from build123d import *

# Parameters (mm, degrees)
SKETCH1_R           = 5.499999036
BOSS_EXTRUDE1_DEPTH = 19
SKETCH2_W           = 11
SKETCH2_H           = 19
CUT_EXTRUDE1_DEPTH  = 33
SKETCH3_W           = 7.598245287
SKETCH3_H           = 4.916511656
CUT_EXTRUDE2_DEPTH  = 33


with BuildPart() as part:
    # Sketch1 → Boss-Extrude1 (new body)
    with BuildSketch(Plane(origin=(0, 0, 0), x_dir=(0, 0, -1), z_dir=(1, 0, 0))):
        with BuildLine():
            Line((-1.999999523, 9.000000954), (11.000000477, 9.000000954))
            Line((11.000000477, 9.000000954), (11.000000477, -9.000000954))
            Line((11.000000477, -9.000000954), (-1.999999523, -9.000000954))
            ThreePointArc((-1.999999523, -9.000000954), (-11.000000477, 0), (-1.999999523, 9.000000954))
        make_face()
        with Locations((-1.999999523, 0)):
            Circle(SKETCH1_R, mode=Mode.SUBTRACT)
    extrude(amount=BOSS_EXTRUDE1_DEPTH)

    # Sketch2 → Cut-Extrude1 (cut)
    with BuildSketch(Plane(origin=(0, 9.000000954, 0), x_dir=(1, 0, 0), z_dir=(0, 1, 0))):
        with Locations((9.5, -1.500000477)):
            Rectangle(SKETCH2_W, SKETCH2_H)
    extrude(amount=-CUT_EXTRUDE1_DEPTH, mode=Mode.SUBTRACT)

    # Sketch3 → Cut-Extrude2 (cut)
    with BuildSketch(Plane.XY.offset(-7.999999523)):
        with Locations((9.476309149, -0.011845426)):
            Rectangle(SKETCH3_W, SKETCH3_H)
    extrude(amount=-CUT_EXTRUDE2_DEPTH, mode=Mode.SUBTRACT)


solid = part.part
Read the model definition and answer for the solid it produces. Units are mm, in the model's axes. A direction names the side the tool comes from. Coordinates: 2 decimals unless noted, no trailing zeros. Order: outer loops, then holes, each group sorted by start corner. A loop starts at its lowest first (then second) coordinate and runs counter-clockwise, first axis right, second up. Notation, with made-up numbers: M 77.5,17 L 117.5,17 A7 ccw 117.5,22 Z; hole C 28,35 d8. An arc over 180 degrees is marked long. Put each result on its own line as item: value. Start each with the question number.
Item 1: Section D-D, the plane y = 5 is taken. Determine the outline of the cut face in (x, z).
Item 2: Given pin 1 Ø6 at (x, y) = (15.5, 4.5) entering from +Z, flat-ended and moving along its own axis, determine where the tip first touches the part or whether it passes through.
Item 3: Consider probe 1 along X at (y, z) = (-1.75, 7.5); probe 2 along Z at (x, y) = (1.9, 0); probe 3 along Y at (x, z) = (15.8, 2). Determine where each line is inside the solid, lowest interval first. Write a range as [from, to].
Item 4: For faces 1 (the face through (9, 9, -9)), 2 (the face through (9, 2.446, -9)), 3 (the face through (9, 4, -8)), determine the directions among +Z, -Z, +X, -X, +Y, -Y from which every point of the face is accessible in a straight line to the end or side of a thin tool.
Item 5: Section A-A, the plane y = 0 is taken. Determine the outline of the cut face in (x, z), plus the area to 3 significant figures.
Item 6: Section B-B, the plane x = 6.5 is taken. Determine the outline of the cut face in (y, z).
Item 7: Section C-C, the plane z = -7 is taken. Determine the outline of the cut face in (x, y), plus the area to 3 significant figures.
Item 8: The mould has two halves that part along X. Classify faces 4 (the face through (5.677, 0, -9)), 5 (the face through (2, 0, 11)), 6 (the face through (0, 0, -5)), 7 (the face through (13.275, 0, -9)): +X half, -X half, draft (parallel to the pull), parting line (faces both ways), or undercut.
Computed:
1. outline: M 0,-11 L 19,-11 L 19,-0.29 L 15,-0.29 L 15,-8 L 4,-8 L 4,-0.29 L 0,-0.29 Z; M 0,4.29 L 4,4.29 L 4,9.48 L 0,9.48 Z; M 15,4.29 L 19,4.29 L 19,9.48 L 15,9.48 Z
2. pin 1: stops at z = 10.87
3. probe 1: x = [0, 4], [15, 19]
3. probe 2: z = [-11, -3.5], [7.5, 11]
3. probe 3: y = [-9, -5.5], [5.5, 9]
4. face 1: +Z, -Z, +X, -X, +Y
4. face 2: +Z, -Z
4. face 3: +Z, +Y, -Y
5. outline: M 0,-11 L 5.68,-11 L 5.68,-8 L 4,-8 L 4,-3.5 L 0,-3.5 Z; M 0,7.5 L 4,7.5 L 4,11 L 0,11 Z; M 13.28,-11 L 19,-11 L 19,-3.5 L 15,-3.5 L 15,-8 L 13.28,-8 Z; M 15,7.5 L 19,7.5 L 19,11 L 15,11 Z
5. area: 98.2 mm2
6. outline: M -9,-11 L -2.47,-11 L -2.47,-8 L -9,-8 Z; M 2.45,-11 L 9,-11 L 9,-8 L 2.45,-8 Z
7. outline: M 0,-9 L 4,-9 L 4,9 L 0,9 Z; M 15,-9 L 19,-9 L 19,9 L 15,9 Z
7. area: 144 mm2
8. face 4: undercut
8. face 5: draft
8. face 6: -X half
8. face 7: undercut
